Autodesk Inventor part; units mm, degrees
ref_plane "YZ Plane" through (0, 0, 0) normal (1, 0, 0) x (0, 1, 0)
ref_plane "XZ Plane" through (0, 0, 0) normal (0, 1, 0) x (-1, 0, 0)
ref_plane "XY Plane" through (0, 0, 0) normal (0, 0, 1) x (1, 0, 0)
sketch "Sketch1" plane through (0, 0, 0) normal (0, 0, 1) x (1, 0, 0)
  line L0 (-9, 22.5) -> (9, 22.5)
  line L1 (9, 22.5) -> (9, -22.5)
  line L2 (9, -22.5) -> (-9, -22.5)
  line L3 (-9, -22.5) -> (-9, 22.5)
  point P0 (0, 0)
  point P1 (0, 22.5)
  point P2 (-9, 0)
  dimension "d0" = 18
  dimension "d1" = 45
extrude "Extrusion1" add sketch "Sketch1" along normal blind 30
sketch "Sketch3" plane through (0, 0, 0) normal (0, 0, -1) x (-1, 0, 0)
  circle A0 centre (-2.5, 0) radius 5.4
  line L0 (-9, -22.5) -> (-9, 22.5)
  point P0 (-9, 0)
  dimension "d4" = 10.8
  dimension "d5" = 6.5
extrude "Extrusion2" cut sketch "Sketch3" against normal through all
sketch "Sketch4" plane through (9, -22.5, 0) normal (1, 0, 0) x (0, 0, -1)
  circle A0 centre (-7, 40) radius 2.75
  circle A1 centre (-7, 5) radius 2.75
  line L0 (0, 0) -> (0, 45)
  line L1 (0, 45) -> (-30, 45)
  line L2 (0, 0) -> (-30, 0)
  circle A2 centre (-23, 40) radius 2.75
  circle A3 centre (-23, 5) radius 2.75
  line L3 (-30, 0) -> (-30, 45)
  point P0 (0, 22.5)
  dimension "d8" = 5.5
  dimension "d9" = 5.5
  dimension "d10" = 7
  dimension "d11" = 5
  dimension "d12" = 5
  dimension "d13" = 7
  dimension "d16" = 35
  dimension "d17" = 16
extrude "Extrusion3" cut sketch "Sketch4" against normal through all contours A1
pattern_linear "Rectangular Pattern1" count 2 spacing 16 along (0, 0, 1) count 2 spacing 35 along (0, 1, 0) of "Extrusion3"
sketch "Sketch5" plane through (-9, -22.5, 0) normal (0, -1, 0) x (1, 0, 0)
  line L0 (0, 0) -> (0, 30)
  line L1 (0, 0) -> (18, 0)
  point P0 (12.5, 15)
  point P1 (0, 15)
  point P2 (9, 0)
  dimension "d38" = 12.5
hole "Hole1" at (3.5, -22.5, 15) direction (0, 1, 0) diameter 4.134 end through all
equation "\"d13\" = d10"
properties part number "0005-10-015 suport tija" material "Wood (Maple)"
Design review of the part built by this model. Coordinates are the model's own, in mm. Coordinates: 2 decimals unless noted, no trailing zeros. Order: outer loops, then holes, each group sorted by start corner. A loop starts at its lowest first (then second) coordinate and runs counter-clockwise, first axis right, second up.
Item 1: Take a section at C-C, the plane x = -1.75. Write out the cut boundary in (y, z).
Item 2: Take a section at D-D, the plane y = 0. Write out the cut boundary in (x, z).
Item 3: The part is to be moulded in two halves that separate along Y. For faces 1 (the cylindrical face through (0.13, -16.67, 4.38)), 2 (the flat face through (-4, 0, 30)), 3 (the flat face through (0, -22.5, 15)), say which applies: pulls with the +Y half, pulls with the -Y half, needs draft (parallel to the pull), parting line crosses it, or undercut.
Item 4: For line 1 (X direction, y = 12, z = 15); line 2 (Z direction, x = 3.5, y = 13.5); line 3 (Y direction, x = 6.75, z = 21), list the stretches that pass through material, from the lowest coordinate up.
Item 5: Take a section at B-B, the plane y = -17. Write out the cut boundary in (x, z).
Item 6: Take a section at A-A, the plane z = 23. Write out the cut boundary in (x, y).
The answers:
1. outline: (-22.5, 0) - (-3.33, 0) - (-3.33, 30) - (-22.5, 30) - close; (3.33, 0) - (22.5, 0) - (22.5, 30) - (3.33, 30) - close; hole circle Ø5.5 at (-17.5, 7); hole circle Ø5.5 at (-17.5, 23); hole circle Ø5.5 at (17.5, 7); hole circle Ø5.5 at (17.5, 23)
2. outline: (-9, 0) - (-2.9, 0) - (-2.9, 30) - (-9, 30) - close; (7.9, 0) - (9, 0) - (9, 30) - (7.9, 30) - close
3. face 1: undercut
3. face 2: needs draft
3. face 3: pulls with the -Y half
4. line 1: x = -9 to 1.43, 5.57 to 9
4. line 2: z = 0 to 12.93, 17.07 to 30
4. line 3: y = -22.5 to -19.39, -15.61 to -3.33, 3.33 to 15.61, 19.39 to 22.5
5. outline: (-9, 0) - (9, 0) - (9, 4.3) - (-9, 4.3) - close; (-9, 9.7) - (9, 9.7) - (9, 20.3) - (-9, 20.3) - close; (-9, 25.7) - (9, 25.7) - (9, 30) - (-9, 30) - close; hole circle Ø4.13 at (3.5, 15)
6. outline: (-9, -22.5) - (9, -22.5) - (9, -20.25) - (-9, -20.25) - close; (-9, -14.75) - (9, -14.75) - (9, 14.75) - (-9, 14.75) - close; (-9, 20.25) - (9, 20.25) - (9, 22.5) - (-9, 22.5) - close; hole circle Ø10.8 at (2.5, 0)
